The drawing under review shows one solid part. Ordinate dimensions are in mm from its lowest x, y, z. A direction names the side the tool comes from. Coordinates: 2 decimals unless noted, no trailing zeros. Write each loop counter-clockwise with the first axis right and the second up, starting at its lowest first coordinate (ties: lowest second). Pieces come first, ordered by that corner, then holes.
Q1. Machinability: for the marked faces 4 and 5, which of the approach directions +Z, -Z, +X, -X, +Y, -Y give a long, thin tool a straight path to every point of the face, cutting with its end or side? Answer none if there is none.
Q2. Clearance check with flat-ended pins moving along their axes: pin 1 Ø5.5 at (y, z) = (45.5, 2) entering from +X; pin 2 Ø4 at (y, z) = (71.5, 9.5) entering from +X; pin 3 Ø4 at (x, y) = (57, 46) entering from -Z; pin 4 Ø8 at (x, z) = (37.5, 2) entering from -Y. State where each tip first meets the part, or that it passes through.
Q3. Add section B-B, the plane y = 60. Give the boundary of the cut face in (x, z).
Q4. The part is to be moulded in two halves that separate along Y. For the marked faces 1, 2 and 3, say which applies: +Y half, -Y half, draft (parallel to the pull), parting line (faces both ways), or undercut.
Q5. Add section A-A, the plane x = 60. Give the boundary of the cut face in (y, z).
Q6. Add section D-D, the plane z = 10. Give the boundary of the cut face in (x, y).
Q7. Add section C-C, the plane z = 2. Give the boundary of the cut face in (x, y).
Q8. To check wall thickness, follow probe 1 along Y at (x, z) = (60, 8.25); probe 2 along Z at (x, y) = (90, 20); probe 3 along X at (y, z) = (38.5, 12) (1 decimal). State the ranges of each line that lie inside material, in increasing order.
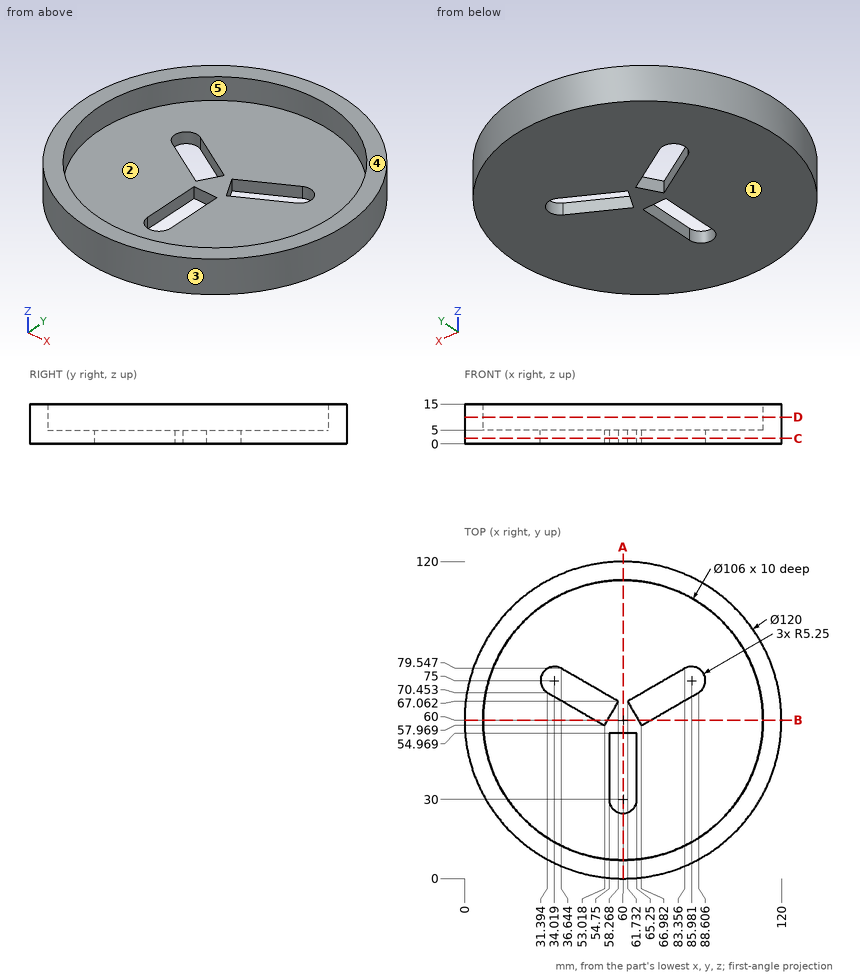
Here are the results:
1. face 4: +Z, +X, -X, +Y, -Y
1. face 5: +Z
2. pin 1: stops at x = 118.84
2. pin 2: stops at x = 119.24
2. pin 3: passes through
2. pin 4: stops at y = 2.92
3. outline: (0, 0) - (49.5, 0) - (49.5, 5) - (7, 5) - (7, 15) - (0, 15) - close; (54.19, 0) - (65.81, 0) - (65.81, 5) - (54.19, 5) - close; (70.5, 0) - (120, 0) - (120, 15) - (113, 15) - (113, 5) - (70.5, 5) - close
4. face 1: draft
4. face 2: undercut
4. face 3: parting line
5. outline: (0, 0) - (24.75, 0) - (24.75, 5) - (7, 5) - (7, 15) - (0, 15) - close; (54.97, 0) - (120, 0) - (120, 15) - (113, 15) - (113, 5) - (54.97, 5) - close
6. outline: circle Ø120 at (60, 60); hole circle Ø106 at (60, 60)
7. outline: circle Ø120 at (60, 60); hole (31.39, 70.45) - (53.02, 57.97) - (58.27, 67.06) - (36.64, 79.55) arc R5.25 ccw to start; hole (54.75, 30) arc R5.25 ccw to (65.25, 30) - (65.25, 54.97) - (54.75, 54.97) - close; hole (61.73, 67.06) - (66.98, 57.97) - (88.61, 70.45) arc R5.25 ccw to (83.36, 79.55) - close
8. probe 1: y = 0 to 7, 113 to 120
8. probe 2: z = 0 to 5
8. probe 3: x = 4 to 11.6, 108.4 to 116
